Verification items for the finished model (mm, model axes). Face numbers are marked on the shaded views. A direction names the side the tool comes from. Coordinates: 2 decimals unless noted, no trailing zeros. Write each loop counter-clockwise with the first axis right and the second up, starting at its lowest first coordinate (ties: lowest second). Pieces come first, ordered by that corner, then holes. Notation, with made-up numbers: (5, 86.25) -> (19, 86.25) arc R24 cw to (19, 105.25) -> close; hole circle Ø11 at (-17.5, -2). An arc over 180 degrees is marked (long way). Use CSV: the item, a comma, the result in double quotes.
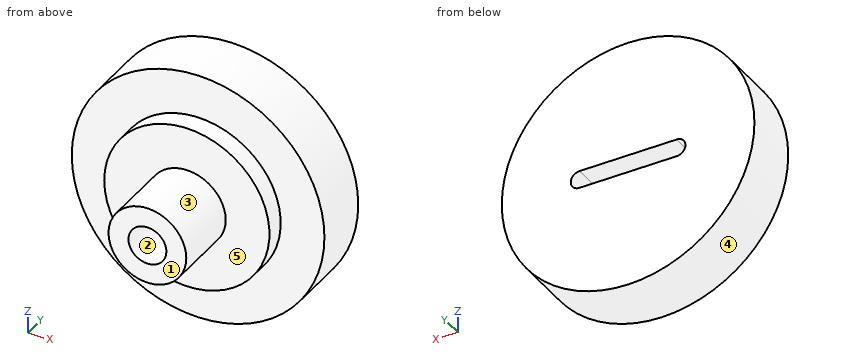
Autodesk Inventor part; units mm, degrees
ref_plane "YZ Plane" through (0, 0, 0) normal (1, 0, 0) x (0, 1, 0)
ref_plane "XZ Plane" through (0, 0, 0) normal (0, 1, 0) x (-1, 0, 0)
ref_plane "XY Plane" through (0, 0, 0) normal (0, 0, 1) x (1, 0, 0)
sketch "Sketch1" plane through (0, 0, 0) normal (0, 1, 0) x (-1, 0, 0)
  circle A0 centre (0, 0) radius 8.5
  dimension "d0" = 17
extrude "Extrusion1" add sketch "Sketch1" along normal blind 2
sketch "Sketch2" plane through (0, 2, 0) normal (0, 1, 0) x (1, 0, 0)
  circle A0 centre (0, 0) radius 13
  dimension "d3" = 26
extrude "Extrusion2" add sketch "Sketch2" along normal blind 6
sketch "Sketch3" plane through (0, 0, 0) normal (0, -1, 0) x (1, 0, 0)
  circle A0 centre (0, 0) radius 4
  dimension "d6" = 8
extrude "Extrusion3" add sketch "Sketch3" along normal blind 7
sketch "Sketch4" plane through (0, -7, 0) normal (0, -1, 0) x (1, 0, 0)
  point P0 (0, 0)
  point P1 (0, 0)
hole "Hole1" at (0, -7, 0) direction (0, 1, 0) diameter 3.9 depth 10 tip angle 118
sketch "Sketch6" plane through (0, 8, 0) normal (0, 1, 0) x (1, 0, 0)
  line L0 (5, 0) -> (-5, 0) construction
  line L1 (5, 0.9) -> (-5, 0.9)
  line L2 (-5, -0.9) -> (5, -0.9)
  arc A0 (5, -0.9) -> (5, 0.9) centre (5, 0) ccw
  arc A1 (-5, 0.9) -> (-5, -0.9) centre (-5, 0) ccw
  point P0 (0, 0)
  point P1 (0, 0)
  dimension "d24" = 1.8
  dimension "d25" = 10
extrude "Extrusion5" cut sketch "Sketch6" against normal blind 5
sketch "Sketch7" plane through (0, 8, 0) normal (0, 1, 0) x (1, 0, 0)
  line L0 (0.9699, -12.5028) -> (-0.9699, -12.5028)
  line L1 (-0.9699, -12.5028) -> (-0.9699, -13.4972)
  line L2 (-0.9699, -13.4972) -> (0.9699, -13.4972)
  line L3 (0.9699, -13.4972) -> (0.9699, -12.5028)
  circle A0 centre (0, 0) radius 13
  line L4 (0.9699, -12.5028) -> (-0.9699, -13.4972) construction
  line L5 (-0.9699, -12.5028) -> (0.9699, -13.4972) construction
  circle A1 centre (0, 0) radius 13
  line L6 (0, -13) -> (0, 0) construction
properties part number "Arm - 608 bearing cap [Med]"
1) Gauge pin test, flat ends, axial feed: pin 1 (3 mm diameter, centred on x = -8, y = 1.5, fed in from -Z); pin 2 (1.5 mm diameter, centred on y = -0.5, z = -3, fed in from +X); pin 3 (1.4 mm diameter, centred on x = 3.5, z = 0, fed in from +Y). Record the tip position at first contact, or that the pin passes through.
Return value:
pin 1,"z = -11.21"
pin 2,"x = 8.14"
pin 3,"y = 3"
2) Cross-section at C-C (y = 5.5). Record the boundary of the cut face in (x, z), plus the area to 3 significant figures.
Return value:
outline,"circle Ø26 at (0, 0); hole (-5, -0.9) -> (5, -0.9) arc R0.9 ccw to (5, 0.9) -> (-5, 0.9) arc R0.9 ccw to start"
area,"510 mm2"
3) Scan lines: L1, parallel to Z at x = 0, y = -3; L2, parallel to X at y = -0.75, z = -1.5; L3, parallel to Z at x = -2.5, y = 4. Record each from-to range of solid material in increasing order.
Return value:
L1,"-4 to -1.95, 1.95 to 4"
L2,"-3.71 to -1.25, 1.25 to 3.71"
L3,"-12.76 to -0.9, 0.9 to 12.76"
4) Cross-section at A-A (x = 0). Record the boundary of the cut face in (y, z).
Return value:
outline,"(-7, -4) -> (0, -4) -> (0, -8.5) -> (2, -8.5) -> (2, -13) -> (8, -13) -> (8, -0.9) -> (3.63, -0.9) -> (3, -1.95) -> (-7, -1.95) -> close; (-7, 1.95) -> (3, 1.95) -> (3.63, 0.9) -> (8, 0.9) -> (8, 13) -> (2, 13) -> (2, 8.5) -> (0, 8.5) -> (0, 4) -> (-7, 4) -> close"
5) Mould release check, pull along Z, two halves, no side actions. Record for the marked faces 1, 2 and 3: released by +Z, released by -Z, zero draft, split by the parting line, or undercut.
Return value:
face 1,"zero draft"
face 2,"undercut"
face 3,"split by the parting line"
6) Set-up check for the marked faces 4 and 5: record each of +Z, -Z, +X, -X, +Y, -Y from which the full face is reachable in a straight line by a thin tool's end or side.
Return value:
face 4,"+Y, -Y"
face 5,"-Y"
7) Cross-section at D-D (z = 6.5). Record the boundary of the cut face in (x, y).
Return value:
outline,"(-11.26, 2) -> (-5.48, 2) -> (-5.48, 0) -> (5.48, 0) -> (5.48, 2) -> (11.26, 2) -> (11.26, 8) -> (-11.26, 8) -> close"
8) Cross-section at B-B (z = 0). Record the boundary of the cut face in (x, y).
Return value:
outline,"(-13, 2) -> (-8.5, 2) -> (-8.5, 0) -> (-4, 0) -> (-4, -7) -> (-1.95, -7) -> (-1.95, 3) -> (-5.9, 3) -> (-5.9, 8) -> (-13, 8) -> close; (1.95, -7) -> (4, -7) -> (4, 0) -> (8.5, 0) -> (8.5, 2) -> (13, 2) -> (13, 8) -> (5.9, 8) -> (5.9, 3) -> (1.95, 3) -> close"
